Geometry: final body of the model. Coordinates: model frame, mm. Face numbers are marked on the shaded views. A direction names the side the tool comes from. Coordinates: 2 decimals unless noted, no trailing zeros. Write each loop counter-clockwise with the first axis right and the second up, starting at its lowest first coordinate (ties: lowest second). Pieces come first, ordered by that corner, then holes. Notation, with made-up numbers: (-21.5, -24) - (-9.5, -24) arc R25 ccw to (-9.5, 1) - close; hole circle Ø10 at (59.5, 24.5). An arc over 180 degrees is marked (long way). Put each result on its own line as item: value.
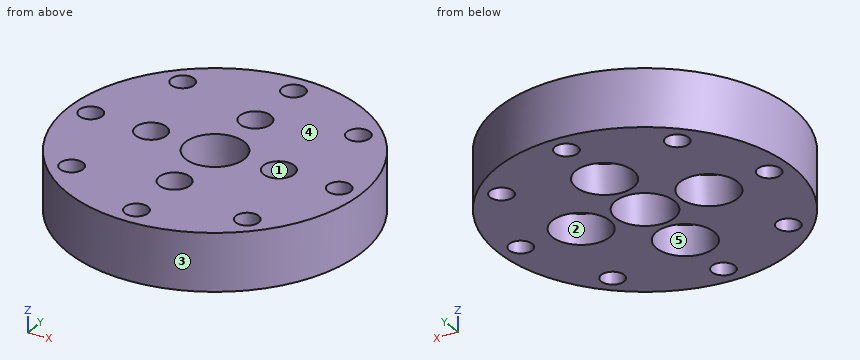
Autodesk Inventor part; units mm, degrees
ref_plane "YZ Plane" through (0, 0, 0) normal (1, 0, 0) x (0, 1, 0)
ref_plane "XZ Plane" through (0, 0, 0) normal (0, 1, 0) x (-1, 0, 0)
ref_plane "XY Plane" through (0, 0, 0) normal (0, 0, 1) x (1, 0, 0)
sketch "スケッチ1" plane through (0, 0, 0) normal (0, 0, 1) x (1, 0, 0)
  circle A0 centre (0, 0) radius 20.5
  dimension "d0" = 41
extrude "押し出し1" add sketch "スケッチ1" along normal blind 8
sketch "スケッチ2" plane through (0, 0, 8) normal (0, 0, 1) x (1, 0, 0)
  circle A0 centre (0, 0) radius 17.5
  point P0 (0, 17.5)
  point P1 (-12.3744, 12.3744)
  point P2 (-17.5, 0)
  point P3 (-12.3744, -12.3744)
  point P4 (0, -17.5)
  point P5 (12.3744, -12.3744)
  point P6 (17.5, 0)
  point P7 (12.3744, 12.3744)
  dimension "d3" = 35
  dimension "d6" = 360
hole "穴1" at (0, 17.5, 8) at (-12.3744, 12.3744, 8) at (-17.5, 0, 8) at (-12.3744, -12.3744, 8) at (0, -17.5, 8) at (12.3744, -12.3744, 8) at (17.5, 0, 8) at (12.3744, 12.3744, 8) direction (0, 0, -1) diameter 3.2 end through all
sketch "スケッチ3" plane through (0, 0, 0) normal (0, 0, -1) x (-1, 0, 0)
  circle A0 centre (0, 0) radius 9
  point P0 (0, 9)
  point P1 (-9, 0)
  point P2 (0, -9)
  point P3 (9, 0)
  dimension "d15" = 18
  dimension "d18" = 360
hole "穴2" at (0, 9, 0) at (9, 0, 0) at (0, -9, 0) at (-9, 0, 0) direction (0, 0, 1) diameter 4.3 end through all counterbore diameter 8 counterbore depth 4.2
sketch "スケッチ4" plane through (0, 0, 8) normal (0, 0, 1) x (1, 0, 0)
  circle A0 centre (0, 0) radius 4.1
  dimension "d27" = 8.2
extrude "押し出し2" cut sketch "スケッチ4" against normal through all
properties part number "scara-base10" material "ABS プラスチック"
1. Section query A-A (y = -17). Return loops of the section in (x, z), then the cut area to 3 significant figures.
Answer below:
outline: (-11.46, 0) - (-1.52, 0) - (-1.52, 8) - (-11.46, 8) - close; (1.52, 0) - (11.46, 0) - (11.46, 8) - (1.52, 8) - close
area: 159 mm²
2. Ray query, probe 1 along Y at (x, z) = (0, 5.5); probe 2 along Y at (x, z) = (12.5, 6); probe 3 along X at (y, z) = (-13, 7.75). Return the intervals inside material, ascending. Write a range as from..to.
Answer below:
probe 1: y = -20.5..-19.1, -15.9..-11.15, -6.85..-4.1, 4.1..6.85, 11.15..15.9, 19.1..20.5
probe 2: y = -16.25..-13.97, -10.78..10.78, 13.97..16.25
probe 3: x = -15.85..-13.85, -10.9..10.9, 13.85..15.85
3. Section query C-C (x = 0). Count the separate pieces of the cut face and the enclosed holes in it, then the cut area to 3 significant figures.
Answer below:
separate pieces: 6
enclosed holes: 0
area: 111 mm²
4. Mould query, pull axis X, two halves, no side actions, for the marked faces 3, 4 and 5. Classes: +X half, -X half, draft (parallel to the pull), parting line (faces both ways), or undercut.
Answer below:
face 3: parting line
face 4: draft
face 5: undercut
5. Set-up query: the marked faces 1 and 2. Return all of +Z, -Z, +X, -X, +Y, -Y with unobstructed straight access to the full face (end or side cutting, diameter ignored); none if empty.
Answer below:
face 1: +Z, -Z
face 2: -Z
6. Pin query (flat end, axial travel): pin 1 Ø1 at (y, z) = (-1.5, 3) entering from -X; pin 2 Ø4 at (x, y) = (0, -9) entering from -Z; pin 3 Ø4 at (x, z) = (-1, 6) entering from -Y; pin 4 Ø5 at (x, y) = (0, 9) entering from -Z. Return the tip coordinate at first contact, or that it passes through.
Answer below:
pin 1: stops at x = -20.48
pin 2: passes through
pin 3: stops at y = -20.5
pin 4: stops at z = 4.2
7. Section query D-D (y = -12.5). Return loops of the section in (x, z), then the cut area to 3 significant figures.
Answer below:
outline: (-16.25, 0) - (-13.97, 0) - (-13.97, 8) - (-16.25, 8) - close; (-10.78, 0) - (-1.94, 0) - (-1.94, 4.2) - (1.94, 4.2) - (1.94, 0) - (10.78, 0) - (10.78, 8) - (-10.78, 8) - close; (13.97, 0) - (16.25, 0) - (16.25, 8) - (13.97, 8) - close
area: 193 mm²
8. Section query B-B (x = -13.5). Return loops of the section in (y, z).
Answer below:
outline: (-15.43, 0) - (-13.51, 0) - (-13.51, 8) - (-15.43, 8) - close; (-11.24, 0) - (11.24, 0) - (11.24, 8) - (-11.24, 8) - close; (13.51, 0) - (15.43, 0) - (15.43, 8) - (13.51, 8) - close
